Work out the finished part from the listing and answer in its coordinate system (mm). A direction names the side the tool comes from. Give positions to 0.01 mm unless a question says otherwise; leave off trailing zeros. Order: outer loops, then holes, each group sorted by start corner. A loop starts at its lowest first (then second) coordinate and runs counter-clockwise, first axis right, second up. Notation, with made-up numbers: (-14.75, 71.5) -> (-3.75, 71.5) arc R26 cw to (-3.75, 110.5) -> close; hole circle Ø3 at (62, 8.5). An arc over 180 degrees is marked (long way). Answer as CSV lines item,"result". Start each with the question number.
1. Find the intervals of material crossed by L1, parallel to Z at x = -41, y = -4; L2, parallel to Z at x = -18, y = -23.5; L3, parallel to Z at x = -55, y = 0, in increasing order.
2. For faces 1 (the cylindrical face through (35.959, 51.074, 123.182)), 2 (the flat face through (-100.965, 12.7, -14.4)), 3 (the cylindrical face through (-57.51, -112.44, 71.69)), determine the directions among +Z, -Z, +X, -X, +Y, -Y from which every point of the face is accessible in a straight line to the end or side of a thin tool.
3. Flat-ended cylindrical pins translate along their axes: pin 1 (5 mm diameter, centred on y = 95.5, z = 17, fed in from +X); pin 2 (4 mm diameter, centred on x = 35.5, y = 52.5, fed in from -Z); pin 3 (5 mm diameter, centred on x = 9, y = 102, fed in from +Z). Find the tip coordinate at first contact, or state that the pin passes through.
4. A cutting plane is placed at A-A (x = 21.5). Give the vertices of the cut face in (y, z).
from build123d import *

# Parameters (mm, degrees)
F2_R     = 25.4
F3_SCALE = 0.6


with BuildPart() as f1:
    # F0 (on Front) → F1 (revolve)
    with BuildSketch(Plane.XZ):
        Polygon((111.125, 222.25), (111.125, 241.3), (-111.125, 241.3), (-111.125, 222.25), (-29.2621003771, 222.25), (-5.1864683628, 222.25), align=None)
        Polygon((-98.425, 101.6), (-5.1864683628, 222.25), (-29.2621003771, 222.25), (-122.5006320143, 101.6), align=None)
        Polygon((-28.575, 101.6), (-98.425, 101.6), (-122.5006320143, 101.6), (-168.275, 101.6), (-168.275, 31.75), (-28.575, 31.75), align=None)
    revolve(axis=Axis((-5.1864683628, 0, 0), (1, 0, 0)))

    # F2
    f2_edges = [f1.edges().sort_by_distance(p)[0] for p in [
        (-98.425, 0, -101.6),
        (-5.186468, 0, -222.25),
        (-51.805734, 0, 161.925),
        (-29.2621, 0, -222.25),
        (-122.500632, 0, -101.6),
        (-75.881366, 0, 161.925),
    ]]
    fillet(f2_edges, radius=F2_R)


with BuildPart() as f1_1:
    # F3: moved
    add(f1.part.scale(F3_SCALE))


solid = f1_1.part
Answer sheet:
1,L1,"z = -144.72 to -131.26, -102.94 to -84.09, -68.1 to -18.63, 18.63 to 68.1, 84.09 to 102.94, 131.26 to 144.72"
1,L2,"z = -142.86 to -111.64, -56.25 to 56.25, 111.64 to 142.86"
1,L3,"z = -144.78 to -133.35, -84.9 to -19.05, 19.05 to 84.9, 133.35 to 144.78"
2,face 1,"+X"
2,face 2,"+Z, -Z, -X, +Y, -Y"
2,face 3,"-X"
3,pin 1,"stops at x = -29.27"
3,pin 2,"stops at z = -135.69"
3,pin 3,"stops at z = 105.17"
4,outline,"circle Ø289.56 at (0, 0); hole circle Ø266.7 at (0, 0)"
